Here's the drawing with two shaded views (mm, measured from the low corner). I have some questions. A direction names the side the tool comes from. Coordinates: 2 decimals unless noted, no trailing zeros. Order: outer loops, then holes, each group sorted by start corner. A loop starts at its lowest first (then second) coordinate and runs counter-clockwise, first axis right, second up. Notation, with made-up numbers: (15.5, 77.5) -> (24.5, 77.5) arc R17 ccw to (24.5, 86.5) -> close; hole circle Ø6 at (-35, 2.25). An arc over 180 degrees is marked (long way). Answer as a JSON object with one key per item and string values. Group by question number.
(1) I need wall thicknesses on line 1 (X direction, y = 7.5, z = 3.95); line 2 (Y direction, x = 13.75, z = 3.4); line 3 (Y direction, x = 3.25, z = 4.6). Which ranges of each line are inside material? Lowest first, please.
(2) I want a section at C-C, the plane x = 16.3. List the corners of the cut face in (y, z) for me (3 decimals).
(3) I want a section at D-D, the plane z = 3.05. List the corners of the cut face in (x, y) for me, plus the area to 3 significant figures.
(4) Which directions (+Z, -Z, +X, -X, +Y, -Y) give clear straight access to the entire face, cutting with the end or side of a thin tool? Please do the marked faces 5 and 6.
(5) For pin 1 (2 mm diameter, centred on x = 7.5, z = 3, fed in from -Y); pin 2 (1.5 mm diameter, centred on x = 12.5, z = 1, fed in from +Y), each with a flat end and sliding along its axis, tell me the tip position at first contact or that it passes through.
(6) I want a section at A-A, the plane y = 12.5. List the corners of the cut face in (x, z) for me.
(7) If we mould it in two halves opening along X, with no side actions, what happens to the marked faces 1, 2, 3 and 4? For each: pulls with the +X half, pulls with the -X half, needs draft (parallel to the pull), parting line crosses it, or undercut.
(8) I want a section at B-B, the plane z = 1.63. List the corners of the cut face in (x, y) for me (3 decimals), plus the area to 3 significant figures.
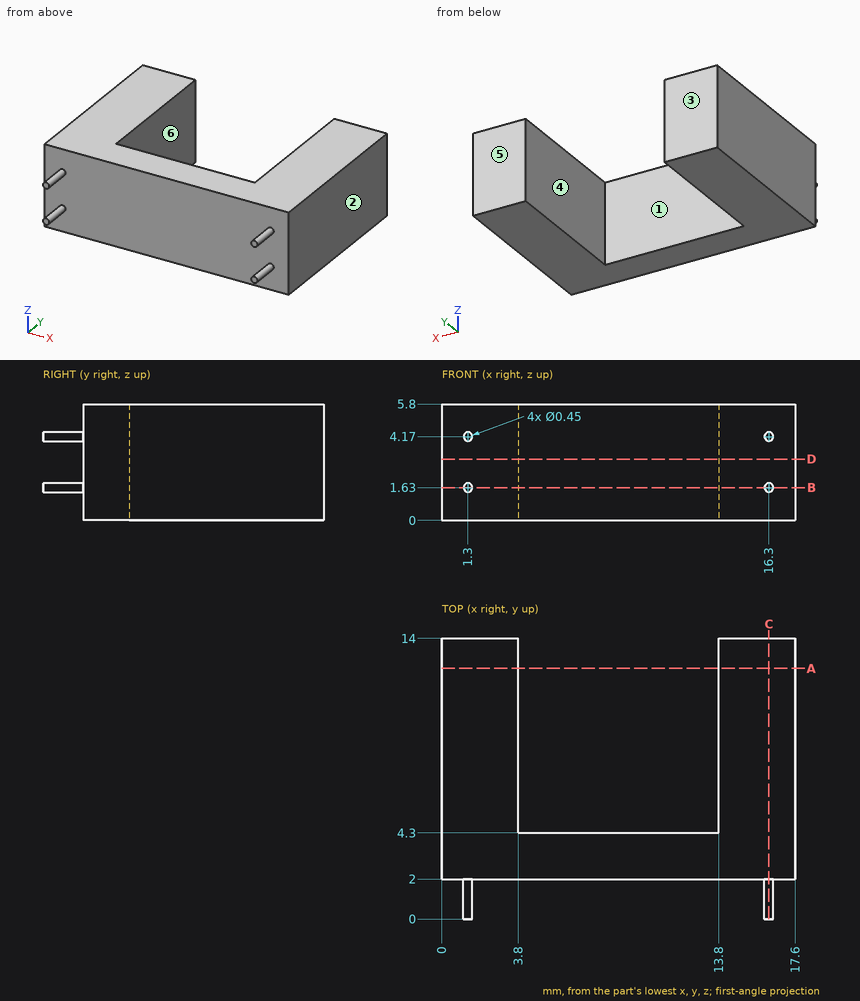
Computed values:
{
 "1": {"line 1": "x = 0 to 3.8, 13.8 to 17.6", "line 2": "y = 2 to 4.3", "line 3": "y = 2 to 14"},
 "2": {"outline": "(0, 1.405) -> (2, 1.405) -> (2, 0) -> (14, 0) -> (14, 5.8) -> (2, 5.8) -> (2, 4.395) -> (0, 4.395) -> (0, 3.945) -> (2, 3.945) -> (2, 1.855) -> (0, 1.855) -> close"},
 "3": {"outline": "(0, 2) -> (17.6, 2) -> (17.6, 14) -> (13.8, 14) -> (13.8, 4.3) -> (3.8, 4.3) -> (3.8, 14) -> (0, 14) -> close", "area": "114 mm2"},
 "4": {"face 5": "+Z, -Z, +X, -X, +Y", "face 6": "+Z, -Z, +Y"},
 "5": {"pin 1": "stops at y = 2", "pin 2": "stops at y = 4.3"},
 "6": {"outline": "(0, 0) -> (3.8, 0) -> (3.8, 5.8) -> (0, 5.8) -> close; (13.8, 0) -> (17.6, 0) -> (17.6, 5.8) -> (13.8, 5.8) -> close"},
 "7": {"face 1": "undercut", "face 2": "pulls with the +X half", "face 3": "needs draft", "face 4": "undercut"},
 "8": {"outline": "(0, 2) -> (1.075, 2) -> (1.075, 0) -> (1.525, 0) -> (1.525, 2) -> (16.075, 2) -> (16.075, 0) -> (16.525, 0) -> (16.525, 2) -> (17.6, 2) -> (17.6, 14) -> (13.8, 14) -> (13.8, 4.3) -> (3.8, 4.3) -> (3.8, 14) -> (0, 14) -> close", "area": "116 mm2"}
}
